```python
from build123d import *

# Parameters (mm, degrees)
SKETCH2_W           = 21.7
SKETCH2_H           = 25.05
SKETCH2_RX          = 9.525
SKETCH2_RY          = 6.35
BOSS_EXTRUDE1_DEPTH = 12.7
SKETCH3_W           = 21.660653916
SKETCH3_H           = 25.05
BOSS_EXTRUDE2_DEPTH = 3
SKETCH5_W           = 18.892037138
SKETCH5_H           = 21.7
BOSS_EXTRUDE3_DEPTH = 2
SKETCH6_W           = 30
SKETCH6_H           = 21.7
BOSS_EXTRUDE4_DEPTH = 4
SKETCH7_W           = 21.7
SKETCH7_H           = 1
SKETCH7_W_2         = 3.175
SKETCH7_H_2         = 3
CUT_EXTRUDE2_DEPTH  = 23
SKETCH7_3_W         = 21.7
SKETCH7_3_H         = 7.272473706
CUT_EXTRUDE3_DEPTH  = 44.803879418
CUT_REVOLVE1_START  = -0.75
CUT_REVOLVE1_DEPTH  = 1.5
FILLET1_R           = 0.6
CUT_EXTRUDE4_REACH  = 47.088
SKETCH9_R           = 1.5
SKETCH10_R          = 2
CUT_EXTRUDE7_DEPTH  = 1
FILLET5_R           = 6.35
FILLET6_R           = 2
FILLET7_R           = 2


# Read off the part's stored shape, not the designer's step: Cut-Revolve1
with BuildPart() as part:
    # Sketch2 → Boss-Extrude1 (new body)
    with BuildSketch(Plane(origin=(16.497783942, 9.525, 0), x_dir=(0, 0, -1), z_dir=(0.8660254037844379, 0.5000000000000013, 0))):
        Rectangle(SKETCH2_W, SKETCH2_H)
        with Locations(Location((0, 0), (0, 0, 90))):
            Ellipse(SKETCH2_RX, SKETCH2_RY, mode=Mode.SUBTRACT)
    extrude(amount=-BOSS_EXTRUDE1_DEPTH)

    # Sketch3 → Boss-Extrude2 (add)
    with BuildSketch(Plane(origin=(5.499261314, 3.175, 0), x_dir=(0, 0, 1), z_dir=(-0.8660254037844379, -0.5000000000000014, 0))):
        with Locations((-0.019673042, 0)):
            Rectangle(SKETCH3_W, SKETCH3_H)
    extrude(amount=BOSS_EXTRUDE2_DEPTH)

    # Sketch5 → Boss-Extrude3 (add)
    with BuildSketch(Plane(origin=(0, 0, 0), x_dir=(-1, 0, 0), z_dir=(0, 1, 0))):
        with Locations((-13.314265373, 0)):
            Rectangle(SKETCH5_W, SKETCH5_H)
    extrude(amount=-BOSS_EXTRUDE3_DEPTH)

    # Sketch6 → Boss-Extrude4 (add)
    with BuildSketch(Plane.XZ.offset(2)):
        with Locations((18.868246804, 0)):
            Rectangle(SKETCH6_W, SKETCH6_H)
    extrude(amount=BOSS_EXTRUDE4_DEPTH)

    # Sketch7 → Cut-Extrude2 (cut)
    with BuildSketch(Plane(origin=(33.868246804, 0, 0), x_dir=(0, 0, -1), z_dir=(1, 0, 0))):
        with Locations((0, -2.5)):
            Rectangle(SKETCH7_W, SKETCH7_H)
        with Locations((0, -4.5)):
            Rectangle(SKETCH7_W_2, SKETCH7_H_2)
    extrude(amount=-CUT_EXTRUDE2_DEPTH, mode=Mode.SUBTRACT)

    # Sketch7<3> → Cut-Extrude3 (cut, through all)
    with BuildSketch(Plane(origin=(33.868246804, 0, 0), x_dir=(0, 0, -1), z_dir=(1, 0, 0))):
        with Locations((0, -9.636236853)):
            Rectangle(SKETCH7_3_W, SKETCH7_3_H)
    extrude(amount=-CUT_EXTRUDE3_DEPTH, mode=Mode.SUBTRACT)

    # Cut-Revolve1 outline → Cut-Revolve1 (cut)
    with BuildSketch(Plane.XY.offset(CUT_REVOLVE1_START)):
        Polygon((6.841174209, 0.850738686), (3.377072594, 0.850738686), (3.868246804, 0), (3.868246804, -5.099015085), (12.7, 0), (7.332348419, 0), align=None)
    extrude(amount=CUT_REVOLVE1_DEPTH, mode=Mode.SUBTRACT)

    # Fillet1
    fillet1_edges = [part.edges().sort_by_distance(p)[0] for p in [
        (5.109123401, 0.850738686, 0.75),
        (5.109123401, 0.850738686, -0.75),
        (8.284123402, -2.549507542, -0.75),
        (8.284123402, -2.549507542, 0.75),
    ]]
    fillet(fillet1_edges, radius=FILLET1_R)

    # Sketch9 → Cut-Extrude4 (cut, up to next)
    with BuildSketch(Plane(origin=(0, 0, -10.85), x_dir=(-1, 0, 0), z_dir=(0, 0, -1)), mode=Mode.PRIVATE) as cut_extrude4_sk1:
        with Locations((-14.332720433, 8.275)):
            Circle(SKETCH9_R)
    cut_extrude4_tool1 = extrude(cut_extrude4_sk1.sketch, amount=-CUT_EXTRUDE4_REACH, mode=Mode.PRIVATE) & part.part
    cut_extrude4 = cut_extrude4_tool1.solids().sort_by_distance((14.33272, 8.275, -10.85))[0]
    add(cut_extrude4, mode=Mode.SUBTRACT)

    # Sketch10 → Cut-Extrude7 (cut)
    with BuildSketch(Plane(origin=(0, 0, -10.85), x_dir=(-1, 0, 0), z_dir=(0, 0, -1))):
        with Locations((-14.332720433, 8.275)):
            Circle(SKETCH10_R)
    cut_extrude7 = extrude(amount=-CUT_EXTRUDE7_DEPTH, mode=Mode.SUBTRACT)

    # Mirror1: Cut-Extrude4, Cut-Extrude7 across plane
    add(cut_extrude4.mirror(Plane.XY), mode=Mode.SUBTRACT)
    add(cut_extrude7.mirror(Plane.XY), mode=Mode.SUBTRACT)

    # Fillet5
    fillet5_edges = [part.edges().sort_by_distance(p)[0] for p in [
        (33.868246804, -4.5, 10.85),
        (33.868246804, -4.5, -10.85),
        (22.760283942, -1, -10.85),
        (22.760283942, -1, 10.85),
        (4.736022628, 17.196968182, 10.85),
        (3.436984522, 16.446968182, -10.85),
    ]]
    fillet(fillet5_edges, radius=FILLET5_R)

    # Fillet6
    fillet6_edges = [part.edges().sort_by_distance(p)[0] for p in [
        (33.868246804, -4.5, 1.5875),
        (33.868246804, -4.5, -1.5875),
    ]]
    fillet(fillet6_edges, radius=FILLET6_R)

    # Fillet7
    # the kernel refuses this fillet: 2 mm, written as the material it takes off along each edge
    with BuildSketch(Plane(origin=(22.760283942, 0, 8.429393602), x_dir=(-1, 0, 0), z_dir=(0, 0, -1))) as fillet7_piece_1:
        with BuildLine():
            CenterArc((2, -1.571757441), FILLET7_R, 128.197977663, 51.802022337)
            Line((0, -1.571757441), (-0.04, -1.571757441))
            Line((-0.04, -1.571757441), (-0.04, 0))
            Line((-0.04, 0), (0, 0.04))
            ThreePointArc((0, 0.04), (0.381619343, 0.04), (0.73850346, 0.031435149))
            Line((0.73850346, 0.031435149), (0.763238686, 0))
        make_face()
    extrude(amount=16.858787203, mode=Mode.SUBTRACT)


solid = part.part
```
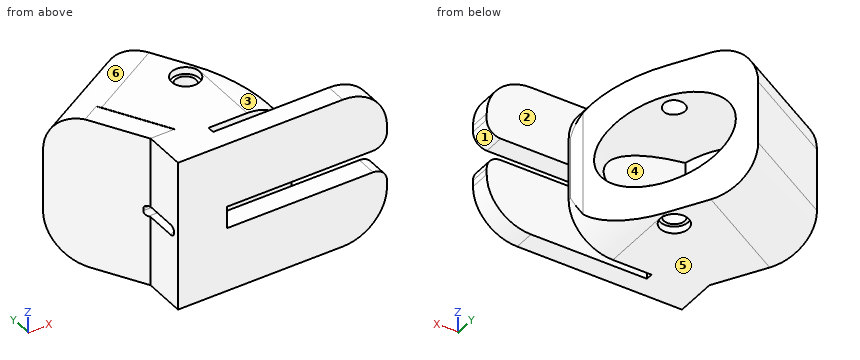
Source: CAD feature listing. Evaluate the final solid. Frame: model axes, mm. Face numbers are marked on the shaded views. A direction names the side the tool comes from. Round coordinates to 2 decimals unless told otherwise and drop trailing zeros. Loops run counter-clockwise (first coordinate to the right, second up) from the corner with the lowest first, then second, coordinate; pieces in that order, holes last.
1. Access query for the marked faces 1, 2 and 3. Directions: +Z, -Z, +X, -X, +Y, -Y. A direction counts if a zero-diameter tool reaches every point of the face in a straight line with its end or side. Return the directions, or none.
2. Ray query, L1, parallel to Y at x = 11, z = -2.25; L2, parallel to Y at x = 22, z = -3.25; L3, parallel to Y at x = 12, z = -4.25. Return the intervals inside material, ascending.
3. Section query B-B on z = 9. Output: boundary loops of the cut face in (x, y) (3 decimals), and give its area (3 significant figures).
4. Section query A-A on x = 24.5. Output: boundary loops of the cut face in (y, z), and give its area (3 significant figures).
5. Section query D-D on x = 20. Give the number of separate pieces and of enclosed holes in the cut face, and give its area (3 significant figures).
6. Mould query, pull axis Z, two halves, no side actions, for the marked faces 4, 5 and 6. Classes: released by +Z, released by -Z, zero draft, split by the parting line, or undercut.
7. Contact query for flat-ended pins moving along their axis: pin 1 (6 mm diameter, centred on x = 23, y = 3.5, fed in from -Z); pin 2 (6 mm diameter, centred on x = 19, z = 5.5, fed in from +Y); pin 3 (3 mm diameter, centred on x = 15, y = 8.5, fed in from -Z); pin 4 (4 mm diameter, centred on x = 2, y = 3.5, fed in from +Z). Output: stop coordinate, or through.
8. Section query C-C on x = 30. Output: boundary loops of the cut face in (y, z), and give its area (3 significant figures).
Answers below:
1. face 1: +X, +Y, -Y
1. face 2: +Z, -Z, +X
1. face 3: +Z, +X, +Y
2. L1: y = -6 to -3, -2 to 0, 16.64 to 19.05
2. L2: y = -6 to -3, -2 to 0
2. L3: y = -6 to -3, -2 to 0, 15.1 to 17.32
3. outline: (-2.426, 10.903) - (3.868, 0) - (3.868, -6) - (31.998, -6) - (31.998, -3) - (10.868, -3) - (10.868, -2) - (20.891, -2) - (20.891, 1.917) - (11.17, 18.753) - close; hole circle Ø3 at (14.333, 8.275)
3. area: 386 mm2
4. outline: (-6, -10.85) - (-3, -10.85) - (-3, -1.59) - (-6, -1.59) - close; (-6, 1.59) - (-3, 1.59) - (-3, 10.85) - (-6, 10.85) - close
4. area: 55.6 mm2
5. separate pieces: 3
5. enclosed holes: 0
5. area: 145 mm2
6. face 4: undercut
6. face 5: released by -Z
6. face 6: released by +Z
7. pin 1: stops at z = -9.74
7. pin 2: stops at y = 10.18
7. pin 3: stops at z = -10.85
7. pin 4: stops at z = 10.81
8. outline: (-6, -10.34) - (-3, -10.34) - (-3, -1.59) - (-6, -1.59) - close; (-6, 1.59) - (-3, 1.59) - (-3, 10.34) - (-6, 10.34) - close
8. area: 52.5 mm2
